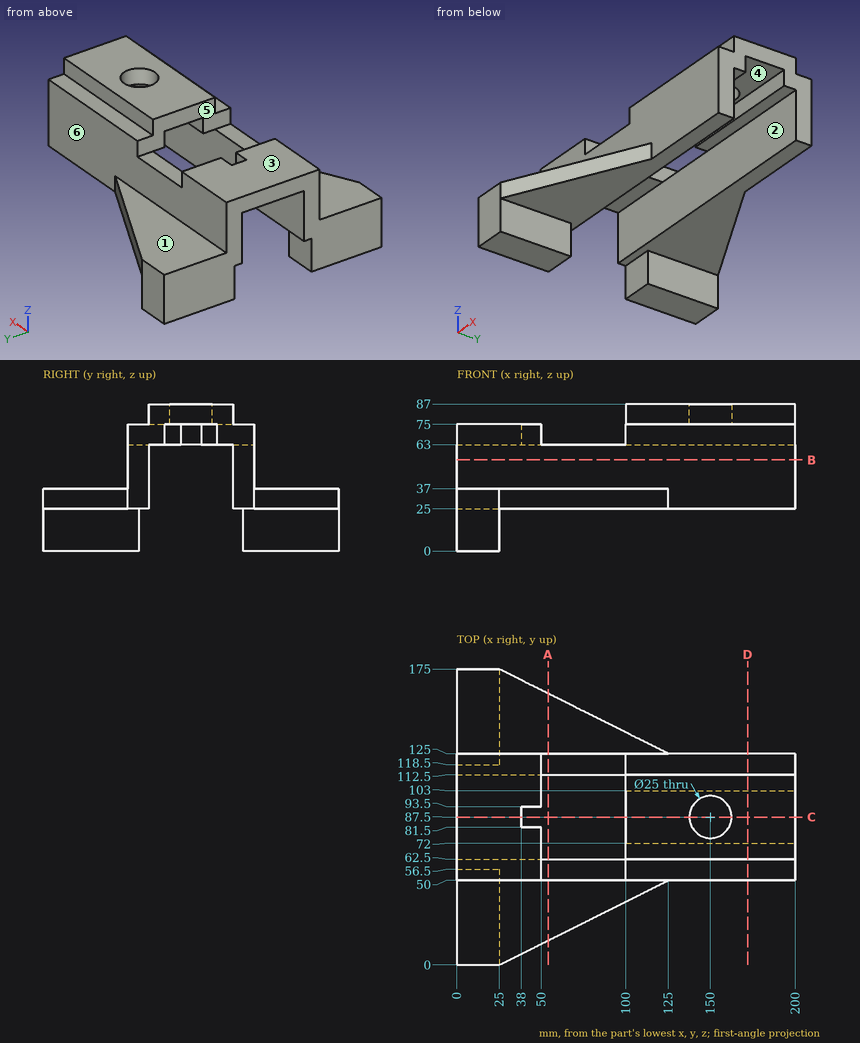
Here's the drawing with two shaded views (mm, measured from the low corner). I have some questions. A direction names the side the tool comes from. Give positions to 0.01 mm unless a question says otherwise; leave off trailing zeros. Loops run counter-clockwise (first coordinate to the right, second up) from the corner with the lowest first, then second, coordinate; pieces in that order, holes last. Notation, with made-up numbers: M 32.25,71.25 L 74.25,71.25 A17 ccw 74.25,91.25 Z; hole C 47.5,-11 d2. An arc over 180 degrees is marked long. Answer in a Markdown table with one row per item.
1. Suppose I cut it at A-A on x = 54. Write out the boundary of the cut face in (y, z), plus the area to 3 significant figures.
Taken from the geometry:
| item | result |
|---|---|
| outline | M 14.5,25 L 62.5,25 L 62.5,63 L 50,63 L 50,37 L 14.5,37 Z; M 112.5,25 L 160.5,25 L 160.5,37 L 125,37 L 125,63 L 112.5,63 Z |
| area | 1,800 mm² |
2. Suppose I cut it at D-D on x = 172. Write out the boundary of the cut face in (y, z), plus the area to 3 significant figures.
Taken from the geometry:
| item | result |
|---|---|
| outline | M 50,25 L 62.5,25 L 62.5,63 L 72,63 L 72,75 L 103,75 L 103,63 L 112.5,63 L 112.5,25 L 125,25 L 125,75 L 112.5,75 L 112.5,87 L 62.5,87 L 62.5,75 L 50,75 Z |
| area | 2,080 mm² |
3. Suppose I cut it at B-B on z = 54. Write out the boundary of the cut face in (x, y), plus the area to 3 significant figures.
Taken from the geometry:
| item | result |
|---|---|
| outline | M 0,50 L 200,50 L 200,62.5 L 0,62.5 Z; M 0,112.5 L 200,112.5 L 200,125 L 0,125 Z |
| area | 5,000 mm² |
4. Suppose I cut it at C-C on y = 87.5. Write out the boundary of the cut face in (x, z), plus the area to 3 significant figures.
Taken from the geometry:
| item | result |
|---|---|
| outline | M 0,63 L 38,63 L 38,75 L 0,75 Z; M 100,75 L 137.5,75 L 137.5,87 L 100,87 Z; M 162.5,75 L 200,75 L 200,87 L 162.5,87 Z |
| area | 1,360 mm² |
5. Which directions (+Z, -Z, +X, -X, +Y, -Y) give clear straight access to the entire face, cutting with the end or side of a thin tool? Please do the marked faces 1, 2 and 3.
Taken from the geometry:
| item | result |
|---|---|
| face 1 | +Z, +X, -X, +Y |
| face 2 | -Z, +X, -X |
| face 3 | +Z, -X, +Y, -Y |
6. For pin 1 Ø6 at (x, y) = (66, 120) entering from +Z; pin 2 Ø10.5 at (x, y) = (167, 106) entering from -Z; pin 3 Ø5 at (y, z) = (135.5, 35) entering from +X; pin 4 Ø14 at (x, y) = (168.5, 117) entering from +Z, each with a flat end and sliding along its axis, tell me the tip position at first contact or that it passes through.
Taken from the geometry:
| item | result |
|---|---|
| pin 1 | stops at z = 63 |
| pin 2 | stops at z = 63 |
| pin 3 | stops at x = 109 |
| pin 4 | stops at z = 87 |
7. Thinking about a two-plate mould opening in Y: for the marked faces 4, 5 and 6, which applies, released by +Y, released by -Y, zero draft, split by the parting line, or undercut?
Taken from the geometry:
| item | result |
|---|---|
| face 4 | undercut |
| face 5 | zero draft |
| face 6 | released by +Y |
8. If I drill on line 1 along Y through (x, z) = (162, 26); line 2 along Y through (x, z) = (150, 82.5); line 3 along X through (y, z) = (24, 10), over which ranges is the centre line in solid material (lowest first)?
Taken from the geometry:
| item | result |
|---|---|
| line 1 | y = 50 to 62.5, 112.5 to 125 |
| line 2 | y = 62.5 to 75, 100 to 112.5 |
| line 3 | x = 0 to 25 |
